```python
from build123d import *

# Parameters (mm, degrees)
CYLINDER323_R     = 1
CYLINDER323_DEPTH = 20
CYLINDER324_R     = 1
CYLINDER324_DEPTH = 20
BOX238_W          = 28
BOX238_H          = 1
BOX238_DEPTH      = 8
BOX237_W          = 21
BOX237_H          = 19
BOX237_DEPTH      = 8


with BuildPart() as zylinder325:
    # Cylinder323 → Cylinder323 (new body)
    with BuildSketch(Plane(origin=(22.5, 23, 30.5), x_dir=(1, 0, 0), z_dir=(0, -1, 0))):
        Circle(CYLINDER323_R)
    extrude(amount=CYLINDER323_DEPTH)


with BuildPart() as fusion215:
    # Cylinder324 → Cylinder324 (new body)
    with BuildSketch(Plane(origin=(-1.5, 23, 30.5), x_dir=(1, 0, 0), z_dir=(0, -1, 0))):
        Circle(CYLINDER324_R)
    extrude(amount=CYLINDER324_DEPTH)

    # Fusion215: union Zylinder325
    add(zylinder325.part)


with BuildPart() as obj1:
    # Box238 → Box238 (new body)
    with BuildSketch(Plane(origin=(-3, 5, 26.5), x_dir=(1, 0, 0), z_dir=(0, 0, 1))):
        with Locations((14, 0.5)):
            Rectangle(BOX238_W, BOX238_H)
    extrude(amount=BOX238_DEPTH)


with BuildPart() as obj2:
    # Box237 → Box237 (new body)
    with BuildSketch(Plane.XY.offset(26.5)):
        with Locations((10.5, 9.5)):
            Rectangle(BOX237_W, BOX237_H)
    extrude(amount=BOX237_DEPTH)

    # Fusion214: union obj1
    add(obj1.part)

    # Cut148: cut Fusion215
    add(fusion215.part, mode=Mode.SUBTRACT)


with BuildPart() as obj2_1:
    # Cut148 placement: moved
    add(obj2.part.moved(Location((19.5, 0, -1.75))))


solid = obj2_1.part
```
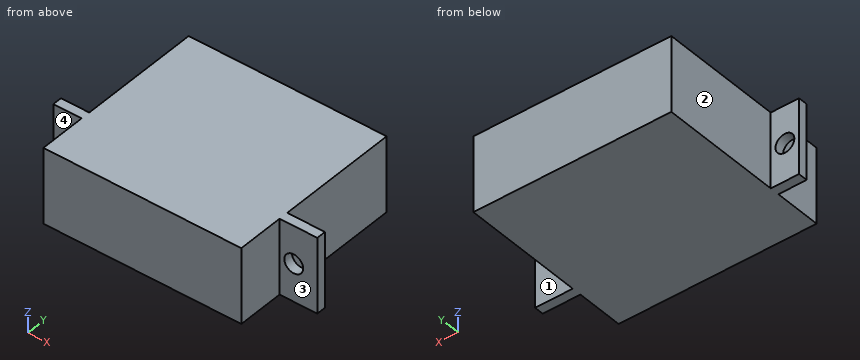
Design review of the part built by this model. Coordinates are the model's own, in mm. Face numbers are marked on the shaded views. A direction names the side the tool comes from. Give positions to 0.01 mm unless a question says otherwise; leave off trailing zeros. Order: outer loops, then holes, each group sorted by start corner. A loop starts at its lowest first (then second) coordinate and runs counter-clockwise, first axis right, second up. Notation, with made-up numbers: (49, 88) -> (61, 88) arc R23 cw to (61, 104) -> close; hole circle Ø4 at (21.25, 4). An arc over 180 degrees is marked (long way). Write item = value, one per line. Start each with the question number.
(1) For pin 1 (0.9 mm diameter, centred on x = 18, z = 29.5, fed in from +Y); pin 2 (1 mm diameter, centred on y = 9, z = 32, fed in from -X); pin 3 (1.5 mm diameter, centred on x = 18.5, z = 29, fed in from -Y); pin 4 (1.8 mm diameter, centred on x = 42, z = 28.75, fed in from +Y), all flat-tipped, find the tip position at first contact; note any pin that passes through.
(2) We need section C-C on z = 26. Write out the cut boundary in (x, y), plus the area to 3 significant figures.
(3) To check wall thickness, follow line 1 along X through (y, z) = (5.65, 28.75); line 2 along Z through (x, y) = (18, 5.35); line 3 along Y through (x, z) = (42, 26.25). State the ranges of each line that lie inside material, in increasing order.
(4) We need section B-B on x = 42. Write out the cut boundary in (y, z), plus the area to 3 significant figures.
(5) For the marked faces 1, 2, 3 and 4, list the 3-axis set-ups (+Z, -Z, +X, -X, +Y, -Y) from which the entire face can be reached by the end or side of a thin tool; tool diameter is ignored.
(6) We need section A-A on z = 28.75. Write out the cut boundary in (x, y), plus the area to 3 significant figures.
(7) We need section D-D on y = 14.75. Write out the cut boundary in (x, z).
Numbers:
q1.pin_1 = 6
q1.pin_2 = 19.5
q1.pin_3 = 5
q1.pin_4 = through
q2.outline = (16.5, 5) -> (19.5, 5) -> (19.5, 0) -> (40.5, 0) -> (40.5, 5) -> (44.5, 5) -> (44.5, 6) -> (40.5, 6) -> (40.5, 19) -> (19.5, 19) -> (19.5, 6) -> (16.5, 6) -> close
q2.area = 406 mm^2
q3.line_1 = 16.5 to 17, 19 to 41, 43 to 44.5
q3.line_2 = 24.75 to 27.75, 29.75 to 32.75
q3.line_3 = 5 to 6
q4.outline = (5, 24.75) -> (6, 24.75) -> (6, 27.75) -> (5, 27.75) -> close; (5, 29.75) -> (6, 29.75) -> (6, 32.75) -> (5, 32.75) -> close
q4.area = 6.00 mm^2
q5.face_1 = +Z, -Z, +X, +Y
q5.face_2 = +Z, -Z, -X, +Y
q5.face_3 = +Z, -Z, +X, -Y
q5.face_4 = +Z, -Z, -X, -Y
q6.outline = (16.5, 5) -> (17, 5) -> (17, 6) -> (16.5, 6) -> close; (19, 5) -> (19.5, 5) -> (19.5, 0) -> (40.5, 0) -> (40.5, 5) -> (41, 5) -> (41, 6) -> (40.5, 6) -> (40.5, 19) -> (19.5, 19) -> (19.5, 6) -> (19, 6) -> close; (43, 5) -> (44.5, 5) -> (44.5, 6) -> (43, 6) -> close
q6.area = 402 mm^2
q7.outline = (19.5, 24.75) -> (40.5, 24.75) -> (40.5, 32.75) -> (19.5, 32.75) -> close
